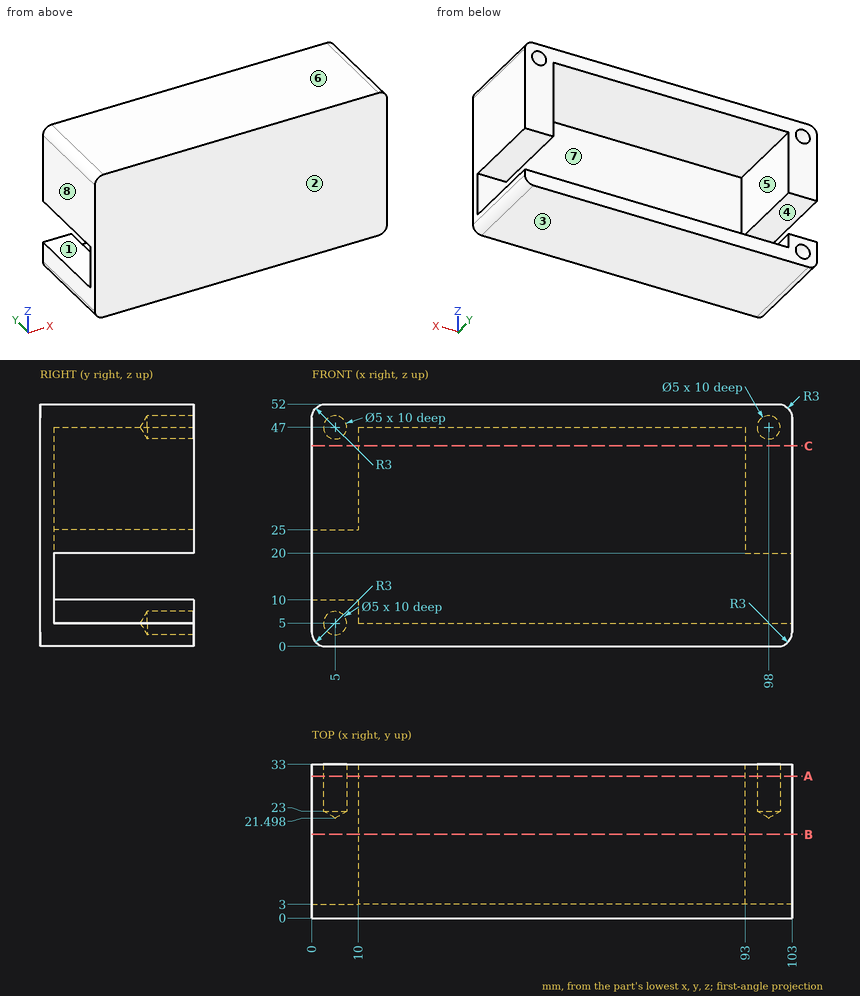
Can you work these out from the drawing? Everything is in mm from the part's minimum corner. A direction names the side the tool comes from. Round coordinates to 2 decimals unless told otherwise and drop trailing zeros. Order: outer loops, then holes, each group sorted by start corner. A loop starts at its lowest first (then second) coordinate and runs counter-clockwise, first axis right, second up.
(1) I'm going to push flat-ended pins straight in: pin 1 (1.5 mm diameter, centred on y = 14, z = 6.5, fed in from +X); pin 2 (5 mm diameter, centred on x = 39, z = 32.5, fed in from +Y); pin 3 (8 mm diameter, centred on y = 13.5, z = 20.5, fed in from -X). Where does each tip first touch, or does it pass through?
Results are:
pin 1: stops at x = 10
pin 2: stops at y = 3
pin 3: stops at x = 93
(2) We'd pull the mould along X, two halves only. Please class the marked faces 6, 7 and 8: +X half, -X half, draft (parallel to the pull), parting line (faces both ways), or undercut.
Results are:
face 6: draft
face 7: undercut
face 8: -X half
(3) If we section it at B-B (y = 18): Please give me the cut outline in (x, z), plus the area to 3 significant figures.
Results are:
outline: (0, 3) arc R3 ccw to (3, 0) - (100, 0) arc R3 ccw to (103, 3) - (103, 5) - (10, 5) - (10, 10) - (0, 10) - close; (0, 25) - (10, 25) - (10, 47) - (93, 47) - (93, 20) - (103, 20) - (103, 49) arc R3 ccw to (100, 52) - (3, 52) arc R3 ccw to (0, 49) - close
area: 1,560 mm2
(4) If we section it at C-C (z = 43): Please give me the cut outline in (x, y), plus the area to 3 significant figures.
Results are:
outline: (0, 0) - (103, 0) - (103, 33) - (93, 33) - (93, 3) - (10, 3) - (10, 33) - (0, 33) - close
area: 909 mm2
(5) On a 3-axis mill with a long thin cutter (end or side, diameter ignored), from which of +Z, -Z, +X, -X, +Y, -Y can I reach the whole of each face in a straight line? I mean the marked faces 1, 2, 3, 4 and 5. Say none if no direction works.
Results are:
face 1: +X, -X, +Y
face 2: +Z, -Z, +X, -X, -Y
face 3: -Z, +X, -X, +Y, -Y
face 4: -X, +Y
face 5: +Y
(6) If we section it at A-A (y = 30.5): Please give me the cut outline in (x, z), plus the area to 3 significant figures.
Results are:
outline: (0, 3) arc R3 ccw to (3, 0) - (100, 0) arc R3 ccw to (103, 3) - (103, 5) - (10, 5) - (10, 10) - (0, 10) - close; (0, 25) - (10, 25) - (10, 47) - (93, 47) - (93, 20) - (103, 20) - (103, 49) arc R3 ccw to (100, 52) - (3, 52) arc R3 ccw to (0, 49) - close; hole circle Ø5 at (5, 5); hole circle Ø5 at (5, 47); hole circle Ø5 at (98, 47)
area: 1,500 mm2
(7) If I drill on L1, parallel to Z at x = 98, y = 28; L2, parallel to Z at x = 28.5, y = 26; L3, parallel to Z at x = 5, y = 26.25, over which ranges is the centre line in solid material (lowest first)?
Results are:
L1: z = 0 to 5, 20 to 44.5, 49.5 to 52
L2: z = 0 to 5, 47 to 52
L3: z = 0 to 2.5, 7.5 to 10, 25 to 44.5, 49.5 to 52
